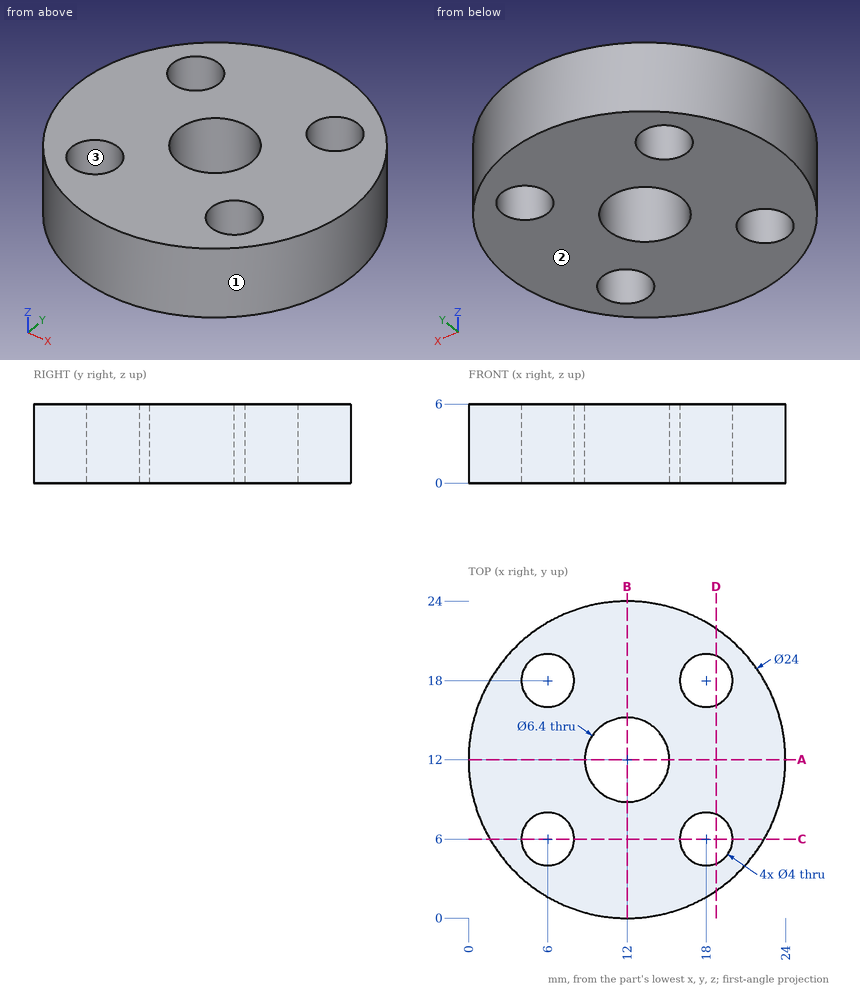
Geometry check sheet. Reference: drawing and pictorial views, mm from the part's lowest x, y, z. Give positions to 0.01 mm unless a question says otherwise; leave off trailing zeros. Order: outer loops, then holes, each group sorted by start corner. A loop starts at its lowest first (then second) coordinate and runs counter-clockwise, first axis right, second up. Notation, with made-up numbers: M 63.5,-32 L 120.5,-32 A9 cw 120.5,-25 Z; hole C 39,-14.5 d8. An arc over 180 degrees is marked long. Return JSON: item names as keys, results as strings. Group by question number.
1) Go/stop test with flat-tipped pins: pin 1 Ø3 at (y, z) = (3.5, 1) entering from +X; pin 2 Ø5 at (x, y) = (18, 6) entering from -Z; pin 3 Ø1 at (y, z) = (10, 2.5) entering from +X; pin 4 Ø1.5 at (x, z) = (3.5, 4) entering from -Y. Record where each tip stops, or that it passes through.
2) Section check D-D on x = 18.75. Record the cut outline in (y, z).
3) Section check C-C on y = 6. Record the cut outline in (x, z).
4) Mould release check, pull along Y, two halves, no side actions. Record for the marked faces 1, 2 and 3: pulls with the +Y half, pulls with the -Y half, needs draft (parallel to the pull), parting line crosses it, or undercut.
5) Scan lines: line 1 (Y direction, x = 6, z = 1.95); line 2 (X direction, y = 5.5, z = 5.6); line 3 (X direction, y = 16.25, z = 4.7). Record each from-to range of solid material in increasing order.
6) Section check A-A on y = 12. Record the cut outline in (x, z).
Answer block:
{
 "1": {"pin 1": "stops at x = 21.75", "pin 2": "stops at z = 0", "pin 3": "stops at x = 23.91", "pin 4": "stops at y = 2.84"},
 "2": {"outline": "M 2.08,0 L 4.15,0 L 4.15,6 L 2.08,6 Z; M 7.85,0 L 16.15,0 L 16.15,6 L 7.85,6 Z; M 19.85,0 L 21.92,0 L 21.92,6 L 19.85,6 Z"},
 "3": {"outline": "M 1.61,0 L 4,0 L 4,6 L 1.61,6 Z; M 8,0 L 16,0 L 16,6 L 8,6 Z; M 20,0 L 22.39,0 L 22.39,6 L 20,6 Z"},
 "4": {"face 1": "parting line crosses it", "face 2": "needs draft", "face 3": "undercut"},
 "5": {"line 1": "y = 1.61 to 4, 8 to 16, 20 to 22.39", "line 2": "x = 1.91 to 4.06, 7.94 to 16.06, 19.94 to 22.09", "line 3": "x = 0.78 to 5.03, 6.97 to 17.03, 18.97 to 23.22"},
 "6": {"outline": "M 0,0 L 8.8,0 L 8.8,6 L 0,6 Z; M 15.2,0 L 24,0 L 24,6 L 15.2,6 Z"}
}
